```python
from build123d import *

# Parameters (mm, degrees)
F1_DEPTH = 63.5
F0_W     = 7.6746088147
F0_H     = 19.05
F2_DEPTH = 25.4
F3_DEPTH = 7.9375
F0_W_2   = 5.0253911853
F0_H_2   = 28.575
F5_R     = 6.35


with BuildPart() as f1:
    # F0 (on Front) → F1 (new body, symmetric)
    with BuildSketch(Plane.XZ):
        Polygon((-41.275, -9.525), (41.275, -9.525), (41.275, 9.525), (22.225, 9.525), (-41.275, 9.525), align=None)
    extrude(amount=F1_DEPTH, both=True)

    # F0 (on Front) → F2 (join, symmetric)
    with BuildSketch(Plane.XZ):
        with BuildLine():
            Line((22.225, 9.525), (41.275, 9.525))
            Line((41.275, 9.525), (41.275, 27.0002))
            ThreePointArc((41.275, 27.0002), (45.9246798487, 38.2255201513), (57.15, 42.8752))
            Line((57.15, 42.8752), (60.325, 42.8752))
            Line((60.325, 42.8752), (60.325, 61.9252))
            Line((60.325, 61.9252), (57.15, 61.9252))
            add(Edge.make_bspline(
                [(57.15, 61.9252), (57.0081649495, 61.9244790011), (56.8664276787, 61.9236160554), (56.7247885758, 61.9226114323)],
                knots=[0, 0, 0, 0, 0.27673231, 0.27673231, 0.27673231, 0.27673231], degree=3))
            ThreePointArc((56.7247885758, 61.9226114323), (32.3044155433, 51.5451090038), (22.225, 27.0002))
            Line((22.225, 27.0002), (22.225, 9.525))
        make_face()
        with Locations((64.1623044074, 52.4002)):
            Rectangle(F0_W, F0_H)
    extrude(amount=F2_DEPTH, both=True)

    # F0 (on Front) → F3 (join, symmetric)
    with BuildSketch(Plane.XZ):
        with BuildLine():
            add(Edge.make_bspline(
                [(56.7247885758, 61.9226114323), (-0.2046186236, 61.5188203951), (-41.275, 38.2270255061), (-41.275, 9.525)],
                knots=[0.27673231, 0.27673231, 0.27673231, 0.27673231, 111.5045361635, 111.5045361635, 111.5045361635, 111.5045361635], degree=3))
            Line((-41.275, 9.525), (22.225, 9.525))
            Line((22.225, 9.525), (22.225, 27.0002))
            ThreePointArc((22.225, 27.0002), (32.3044155433, 51.5451090038), (56.7247885758, 61.9226114323))
        make_face()
    extrude(amount=F3_DEPTH, both=True)

    # F0 (on Front) → F4 (revolve)
    with BuildSketch(Plane.XZ):
        with Locations((108.6123044074, 52.3875)):
            Rectangle(F0_W_2, F0_H_2)
    revolve(axis=Axis((85.725, 0, 52.3875), (0, 0, 1)))

    # F5
    f5_edges = [f1.edges().sort_by_distance(p)[0] for p in [
        (41.275, -63.5, 0),
        (-41.275, -63.5, 0),
        (41.275, 63.5, 0),
        (-41.275, 63.5, 0),
    ]]
    fillet(f5_edges, radius=F5_R)


solid = f1.part
```
Work out the finished part from the listing and answer in its coordinate system (mm). A direction names the side the tool comes from. Give positions to 0.01 mm unless a question says otherwise; leave off trailing zeros. Loops run counter-clockwise (first coordinate to the right, second up) from the corner with the lowest first, then second, coordinate; pieces in that order, holes last. Notation, with made-up numbers: (-0.75, 25.5) -> (48.25, 25.5) arc R23 ccw to (48.25, 35.5) -> close; hole circle Ø2 at (12, 83.25). An arc over 180 degrees is marked (long way). Put each result on its own line as item: value. Start each with the question number.
Item 1: The mould has two halves that part along X. Classify faces 1 (the face through (105.16, 6.12, 52.59)), 2 (the face through (68, 0, 52)), 3 (the face through (40, -25.4, 36)), 4 (the face through (41.275, -1, 4)): released by +X, released by -X, zero draft, split by the parting line, or undercut.
Item 2: Which of the six approach directions +Z, -Z, +X, -X, +Y, -Y give full straight-line access (tool end or side, diameter ignored) to faces 5 (the face through (-4, 7.938, 30)), 6 (the face through (32.57, -16.79, 51.81)), 7 (the face through (60, 0, 61.925)), 8 (the face through (40, 25.4, 36)), 9 (the face through (0, -63.5, 0))?
Item 3: The part is cut by section B-B (z = -1). Give the vertices of the cut face in (x, y) (3 decimals), then the cut area to 3 significant figures.
Item 4: The part is cut by section A-A (x = 93). Give the vertices of the cut face in (y, z) (3 decimals).
Item 5: The part is cut by section C-C (x = 75). Give the vertices of the cut face in (y, z) (3 decimals).
Item 6: Find the intervals of material crossed by L1, parallel to Y at x = 87, z = 49.5; L2, parallel to Y at x = -13.5, z = 34; L3, parallel to X at y = -0.5, z = -0.5 (3 decimals), in increasing order. Write a range as [from, to].
Item 7: Each of these flat-tipped pins is pushed along its axis until it touches: P1, Ø1, axis at y = 5, z = 45, coming from the +X side; P2, Ø2, axis at x = 29, z = 30.5, coming from the -Y side; P3, Ø3, axis at x = 67.5, y = 0.5, coming from the +Z side. Where does it stop, or does it pass through?
Answers below:
1. face 1: undercut
1. face 2: undercut
1. face 3: zero draft
1. face 4: released by +X
2. face 5: +Z, -X, +Y
2. face 6: +Z, -X, -Y
2. face 7: +Z, -X
2. face 8: +Z, +X, -X, +Y
2. face 9: +Z, -Z, +X, -X, -Y
3. outline: (-41.275, -57.15) arc R6.35 ccw to (-34.925, -63.5) -> (34.925, -63.5) arc R6.35 ccw to (41.275, -57.15) -> (41.275, 57.15) arc R6.35 ccw to (34.925, 63.5) -> (-34.925, 63.5) arc R6.35 ccw to (-41.275, 57.15) -> close
3. area: 10,400 mm2
4. outline: (-24.336, 38.1) -> (-19.032, 38.1) -> (-19.032, 66.675) -> (-24.336, 66.675) -> close; (19.032, 38.1) -> (24.336, 38.1) -> (24.336, 66.675) -> (19.032, 66.675) -> close
5. outline: (-23.025, 38.1) -> (-17.323, 38.1) -> (-17.323, 66.675) -> (-23.025, 66.675) -> close; (17.323, 38.1) -> (23.025, 38.1) -> (23.025, 66.675) -> (17.323, 66.675) -> close
6. L1: [-25.37, -20.33], [20.33, 25.37]
6. L2: [-7.94, 7.94]
6. L3: [-41.275, 41.275]
7. P1: x = 110.72
7. P2: y = -25.4
7. P3: z = 61.93
